Could you check a few things on this model? Use its own coordinates, in mm. Give positions to 0.01 mm unless a question says otherwise; leave off trailing zeros. Write each loop counter-clockwise with the first axis right and the second up, starting at its lowest first coordinate (ties: lowest second). Pieces come first, ordered by that corner, then holes. Notation, with made-up numbers: (-36, -10) - (-29, -10) arc R18 ccw to (-29, 22) - close; hole circle Ø11 at (14.25, 9.5). An arc over 180 degrees is marked (long way). Answer as CSV lines item,"result". Start each with the question number.
Q1. Imagine slicing it at A-A on y = 4. List the corners of the cut face in (x, z) for me, and give its area (3 significant figures).
Q2. We'd pull the mould along Z, two halves only. Please class faces 1 (the face through (-19, 0, 27)), 2 (the face through (-2, 9, -5.783)), 3 (the face through (-22.715, 7.148, 21.593)): pulls with the +Z half, pulls with the -Z half, needs draft (parallel to the pull), parting line crosses it, or undercut.
Q3. Imagine slicing it at D-D on y = 11. List the corners of the cut face in (x, z) for me.
Q4. Will these pins go through, and if not, where does the flat tip stop? pin 1 Ø8 at (x, y) = (2, 2) entering from -Z; pin 2 Ø6 at (y, z) = (11, 38.5) entering from -X; pin 3 Ø1.5 at (y, z) = (2.5, 25.5) entering from +X; pin 4 Ø8 at (y, z) = (8, 21.5) entering from +X.
Q5. Imagine slicing it at C-C on x = -28.5. List the corners of the cut face in (y, z) for me.
Q6. Imagine slicing it at B-B on z = 43. List the corners of the cut face in (x, y) for me, and give its area (3 significant figures).
Q7. If I drill on line 1 along X through (y, z) = (14.25, 3); line 2 along Z through (x, y) = (-15.5, 3.25); line 3 along Z through (x, y) = (-16, 5.75), over which ranges is the centre line in solid material (lowest first)?
```python
from build123d import *

# Parameters (mm, degrees)
BOSS_EXTRUDE3_DEPTH                        = 14.5
SKETCH8_R                                  = 6.884606738
CUT_EXTRUDE3_DEPTH                         = 88
F_39_0_21653543_DIAMETER_HOLE1_D           = 5.499999922
F_39_0_21653543_DIAMETER_HOLE1_ON_FACE_2_D = 5.499999922


with BuildPart() as part:
    # Sketch6 → Boss-Extrude3 (new body)
    with BuildSketch(Plane(origin=(0, 0, 0), x_dir=(1, 0, 0), z_dir=(0, 1, 0))):
        Polygon((-16.836914056, 5.783353512), (13.163085944, 5.783353512), (33.163085944, -49.166194877), (-36.836914056, -49.166194877), align=None)
    extrude(amount=BOSS_EXTRUDE3_DEPTH)

    # Sketch8 → Cut-Extrude3 (cut)
    with BuildSketch(Plane.XY.offset(49.166194877)):
        with Locations((-1.836914056, 0)):
            Circle(SKETCH8_R)
    extrude(amount=-CUT_EXTRUDE3_DEPTH, mode=Mode.SUBTRACT)

    # #39 (0.21653543) Diameter Hole1 (through all)
    with Locations(Plane(origin=(17.988085944, 14.5, 24.13287332), x_dir=(0, 0, 1), z_dir=(0, 1, 0))):
        with Locations((0, 0), (18.916226832, 4.825), (18.916226832, -44.475), (-18.916226832, -34.825), (-18.916226832, -4.825), (0, -39.65)):
            Hole(F_39_0_21653543_DIAMETER_HOLE1_D / 2)

    # #39 (0.21653543) Diameter Hole1 on face 2 (through all)
    with Locations(Plane(origin=(-16.836914056, 0, 5.216646488), x_dir=(0, 0, -1), z_dir=(0, -1, 0))):
        with Locations((0, 0), (0, 30), (-37.832453664, 39.65), (-37.832453664, -9.65)):
            Hole(F_39_0_21653543_DIAMETER_HOLE1_ON_FACE_2_D / 2)


solid = part.part
```
Conclusion:
1,outline,"(-36.84, 49.17) - (-16.84, -5.78) - (-7.44, -5.78) - (-7.44, 49.17) - close; (3.77, -5.78) - (13.16, -5.78) - (33.16, 49.17) - (3.77, 49.17) - close; hole circle Ø5.5 at (-26.49, 43.05); hole circle Ø5.5 at (-21.66, 24.13); hole circle Ø5.5 at (-16.84, 5.22); hole circle Ø5.5 at (13.16, 5.22); hole circle Ø5.5 at (17.99, 24.13); hole circle Ø5.5 at (22.81, 43.05)"
1,area,"1,990 mm^2"
2,face 1,"needs draft"
2,face 2,"pulls with the -Z half"
2,face 3,"undercut"
3,outline,"(-36.84, 49.17) - (-16.84, -5.78) - (13.16, -5.78) - (33.16, 49.17) - close; hole circle Ø5.5 at (-26.49, 43.05); hole circle Ø5.5 at (-21.66, 24.13); hole circle Ø5.5 at (-16.84, 5.22); hole circle Ø5.5 at (13.16, 5.22); hole circle Ø5.5 at (17.99, 24.13); hole circle Ø5.5 at (22.81, 43.05)"
4,pin 1,"z = -5.78"
4,pin 2,"x = -34.05"
4,pin 3,"x = 24.82"
4,pin 4,"x = 24.55"
5,outline,"(0, 26.26) - (14.5, 26.26) - (14.5, 41.18) - (0, 41.18) - close; (0, 44.92) - (14.5, 44.92) - (14.5, 49.17) - (0, 49.17) - close"
6,outline,"(-34.59, 0) - (-29.24, 0) - (-29.24, 14.5) - (-34.59, 14.5) - close; (-23.74, 0) - (-8.72, 0) arc R6.88 cw to (5.05, 0) - (20.06, 0) - (20.06, 14.5) - (-23.74, 14.5) - close; (25.56, 0) - (30.92, 0) - (30.92, 14.5) - (25.56, 14.5) - close"
6,area,"716 mm^2"
7,line 1,"-20.03 to -18.46, -15.21 to 11.54, 14.79 to 16.36"
7,line 2,"-5.78 to 2.81, 7.62 to 49.17"
7,line 3,"-5.78 to 2.6, 7.84 to 49.17"
